```python
from build123d import *

# Parameters (mm, degrees)
SKETCH_1_R          = 65.5
EXTRUDE_1_DEPTH     = 3
SKETCH_2_R          = 2.9
EXTRUDE_2_DEPTH     = 4
SKETCH_3_R          = 10.65
CUT_EXTRUDE_1_DEPTH = 94.00032258
SKETCH_4_R          = 1.777177549
EXTRUDE_3_DEPTH     = 26.9
CUT_EXTRUDE_2_DEPTH = 98.917669498


with BuildPart() as part:
    # 草图1 → 凸台-拉伸1 (new body)
    with BuildSketch(Plane.XY):
        Circle(SKETCH_1_R)
    extrude(amount=-EXTRUDE_1_DEPTH)

    # 草图2 → 凸台-拉伸2 (add)
    with BuildSketch(Plane.XY):
        with Locations(Location((-63, 0, 0), (0, 0, 148.88786163))):
            Circle(SKETCH_2_R)
        with Locations(Location((-31.5, 54.559600438, 0), (0, 0, 151.11213837))):
            Circle(SKETCH_2_R)
        with Locations(Location((31.5, 54.559600438, 0), (0, 0, 91.11213837))):
            Circle(SKETCH_2_R)
        with Locations(Location((63, 0, 0), (0, 0, 31.11213837))):
            Circle(SKETCH_2_R)
        with Locations(Location((31.5, -54.559600438, 0), (0, 0, 268.88786163))):
            Circle(SKETCH_2_R)
        with Locations(Location((-31.5, -54.559600438, 0), (0, 0, 208.88786163))):
            Circle(SKETCH_2_R)
    extrude(amount=EXTRUDE_2_DEPTH)

    # 草图3 → 切除-拉伸1 (cut, through all)
    with BuildSketch(Plane.XY):
        Circle(SKETCH_3_R)
    extrude(amount=-CUT_EXTRUDE_1_DEPTH, mode=Mode.SUBTRACT)

    # 草图4 → 凸台-拉伸3 (add)
    with BuildSketch(Plane.XY.offset(4)):
        with Locations((-31.5, 54.559600438)):
            Circle(SKETCH_4_R)
        with Locations((31.5, 54.559600438)):
            Circle(SKETCH_4_R)
        with Locations((63, 0)):
            Circle(SKETCH_4_R)
        with Locations((31.5, -54.559600438)):
            Circle(SKETCH_4_R)
        with Locations((-31.5, -54.559600438)):
            Circle(SKETCH_4_R)
        with Locations((-63, 0)):
            Circle(SKETCH_4_R)
    extrude(amount=EXTRUDE_3_DEPTH)

    # 草图5 → 切除-拉伸2 (cut, through all)
    with BuildSketch(Plane.XY):
        with BuildLine():
            ThreePointArc((22.936143614, 49.18671871), (0, 54.27153933), (-22.936143614, 49.18671871))
            ThreePointArc((-22.936143614, 49.18671871), (-30.965446368, 27.126390699), (-8.905118357, 19.097087944))
            ThreePointArc((-8.905118357, 19.097087944), (0, 21.071305154), (8.905118357, 19.097087944))
            ThreePointArc((8.905118357, 19.097087944), (30.965446368, 27.126390699), (22.936143614, 49.18671871))
        make_face()
        with BuildLine():
            ThreePointArc((12.08600412, -17.260602693), (18.248285555, -10.535652577), (20.991122477, -1.836485251))
            ThreePointArc((20.991122477, -1.836485251), (38.974866642, 13.253667845), (54.065019738, -4.73007632))
            ThreePointArc((54.065019738, -4.73007632), (47.000531763, -27.135769665), (31.128876124, -44.456642389))
            ThreePointArc((31.128876124, -44.456642389), (8.009420274, -40.380058544), (12.08600412, -17.260602693))
        make_face()
        with BuildLine():
            ThreePointArc((-20.991122477, -1.836485251), (-18.248285555, -10.535652577), (-12.08600412, -17.260602693))
            ThreePointArc((-12.08600412, -17.260602693), (-8.009420274, -40.380058544), (-31.128876124, -44.456642389))
            ThreePointArc((-31.128876124, -44.456642389), (-47.000531763, -27.135769665), (-54.065019738, -4.73007632))
            ThreePointArc((-54.065019738, -4.73007632), (-38.974866642, 13.253667845), (-20.991122477, -1.836485251))
        make_face()
    extrude(amount=-CUT_EXTRUDE_2_DEPTH, mode=Mode.SUBTRACT)


solid = part.part
```
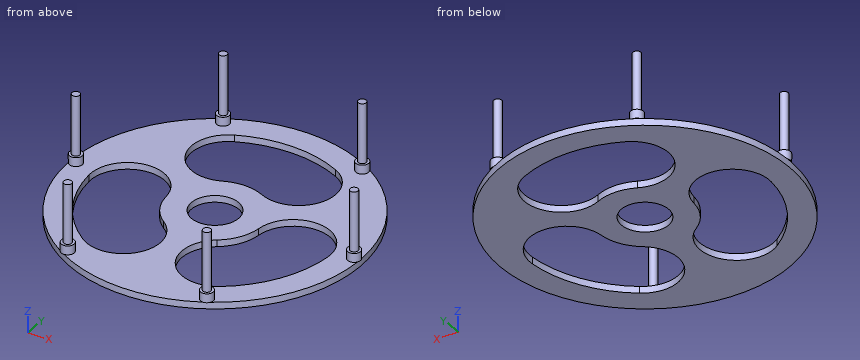
Verification items for the finished model (mm, model axes). Coordinates: 2 decimals unless noted, no trailing zeros. Loops run counter-clockwise (first coordinate to the right, second up) from the corner with the lowest first, then second, coordinate; pieces in that order, holes last. Notation, with made-up numbers: (18, -40) - (42, -40) arc R22 cw to (42, -26) - close; hole circle Ø9 at (15.5, -17). An arc over 180 degrees is marked (long way). Put each result on its own line as item: value.
Item 1: Gauge pin test, flat ends, axial feed: pin 1 Ø10 at (x, z) = (-16.5, 6) entering from -Y; pin 2 Ø0.5 at (x, y) = (-66, 0) entering from -Z; pin 3 Ø24.5 at (x, y) = (0, 0) entering from +Z. Record the tip position at first contact, or that the pin passes through.
Conclusion:
pin 1: passes through
pin 2: stops at z = 0
pin 3: stops at z = 0
Item 2: Section check A-A (x = 0). Enter the section's corners in (y, z), then the cut area to 3 significant figures.
Conclusion:
outline: (-65.5, -3) - (-10.65, -3) - (-10.65, 0) - (-65.5, 0) - close; (10.65, -3) - (21.07, -3) - (21.07, 0) - (10.65, 0) - close; (54.27, -3) - (65.5, -3) - (65.5, 0) - (54.27, 0) - close
area: 229 mm2
Item 3: Section check B-B (y = 27). Enter the section's corners in (x, z).
Conclusion:
outline: (-59.68, -3) - (-30.91, -3) - (-30.91, 0) - (-59.68, 0) - close; (30.91, -3) - (59.68, -3) - (59.68, 0) - (30.91, 0) - close
Item 4: Section check C-C (x = 38). Enter the section's corners in (y, z), then the cut area to 3 significant figures.
Conclusion:
outline: (-53.35, -3) - (-38.75, -3) - (-38.75, 0) - (-53.35, 0) - close; (13.31, -3) - (53.35, -3) - (53.35, 0) - (13.31, 0) - close
area: 164 mm2
Item 5: Section check D-D (y = -30.5). Enter the section's corners in (x, z).
Conclusion:
outline: (-57.97, -3) - (-44.89, -3) - (-44.89, 0) - (-57.97, 0) - close; (-5.01, -3) - (5.01, -3) - (5.01, 0) - (-5.01, 0) - close; (44.89, -3) - (57.97, -3) - (57.97, 0) - (44.89, 0) - close
Item 6: Scan lines: line 1 along Z through (x, y) = (30.5, -51.5); line 2 along X through (y, z) = (-55, 13). Record each from-to range of solid material in increasing order.
Conclusion:
line 1: z = -3 to 0
line 2: x = -33.22 to -29.78, 29.78 to 33.22
